Input: part model. Units: mm. Frame: model coordinates. A direction names the side the tool comes from. Round coordinates to 2 decimals unless told otherwise and drop trailing zeros. Loops run counter-clockwise (first coordinate to the right, second up) from the corner with the lowest first, then second, coordinate; pieces in that order, holes last. Notation, with made-up numbers: M -9,10.5 L 39,10.5 A35 cw 39,48.5 Z; hole C 87,-38.75 d6. An arc over 180 degrees is marked long. Put each result on its own line as item: value. Start each with the question number.
1) Line query: probe 1 along Y at (x, z) = (15.5, -15); probe 2 along X at (y, z) = (32.5, -1); probe 3 along X at (y, z) = (2.5, 15). Output: solid intervals per line, ascending.
2) Reachability of faces 1 (the face through (-4.336, -5.07, 19.524)), 2 (the face through (23.846, -45.49, -7.509)) from +Z, -Z, +X, -X, +Y, -Y: full face, straight path, thin tool, end or side. Return the list, or none.
3) Section C-C on y = 20.5. Output: boundary loops of the cut face in (x, z).
4) Section A-A on x = 0. Output: boundary loops of the cut face in (y, z), plus the area to 3 significant figures.
5) Pin query (flat end, axial travel): pin 1 (4 mm diameter, centred on x = -15.5, y = -59, fed in from +Z); pin 2 (6 mm diameter, centred on x = 15, y = -23, fed in from +Z); pin 3 (1 mm diameter, centred on x = -3.5, y = -61.5, fed in from +Z). Return the tip coordinate at first contact, or that it passes through.
6) Draft query along Y for faces 3 (the face through (-11, -10, -17)), 4 (the face through (23.846, 25.35, -7.509)), 5 (the face through (0, -80, 0)). Return one class per face: +Y half, -Y half, draft (parallel to the pull), parting line (faces both ways), or undercut.
7) Section B-B on z = 0. Output: boundary loops of the cut face in (x, y), plus the area to 3 significant figures.
from build123d import *

# Parameters (mm, degrees)
SKETCH_4_R      = 25
EXTRUDE_1_DEPTH = 50
SKETCH_5_R      = 20
EXTRUDE_2_DEPTH = 50
SKETCH_6_R      = 25
EXTRUDE_3_DEPTH = 70


with BuildPart() as part:
    # 草图4 → 凸台-拉伸1 (new body)
    with BuildSketch(Plane(origin=(0, 50, 0), x_dir=(1, 0, 0), z_dir=(0, 1, 0))):
        Circle(SKETCH_4_R)
    extrude(amount=-EXTRUDE_1_DEPTH)

    # 草图5 → 凸台-拉伸2 (add)
    with BuildSketch(Plane(origin=(0, -10, 0), x_dir=(1, 0, 0), z_dir=(0, 1, 0))):
        Circle(SKETCH_5_R)
    extrude(amount=EXTRUDE_2_DEPTH)

    # 草图6 → 凸台-拉伸3 (add)
    with BuildSketch(Plane(origin=(0, -80, 0), x_dir=(1, 0, 0), z_dir=(0, 1, 0))):
        Circle(SKETCH_6_R)
    extrude(amount=EXTRUDE_3_DEPTH)


solid = part.part
Geometry results:
1. probe 1: y = -80 to -10, 0 to 50
1. probe 2: x = -24.98 to 24.98
1. probe 3: x = -20 to 20
2. face 1: none
2. face 2: +Y, -Y
3. outline: C 0,0 d50
4. outline: M -80,-25 L -10,-25 L -10,-20 L 0,-20 L 0,-25 L 50,-25 L 50,25 L 0,25 L 0,20 L -10,20 L -10,25 L -80,25 Z
4. area: 6,400 mm²
5. pin 1: stops at z = 21.04
5. pin 2: stops at z = 21.93
5. pin 3: stops at z = 24.82
6. face 3: undercut
6. face 4: draft
6. face 5: -Y half
7. outline: M -25,-80 L 25,-80 L 25,-10 L 20,-10 L 20,0 L 25,0 L 25,50 L -25,50 L -25,0 L -20,0 L -20,-10 L -25,-10 Z
7. area: 6,400 mm²
